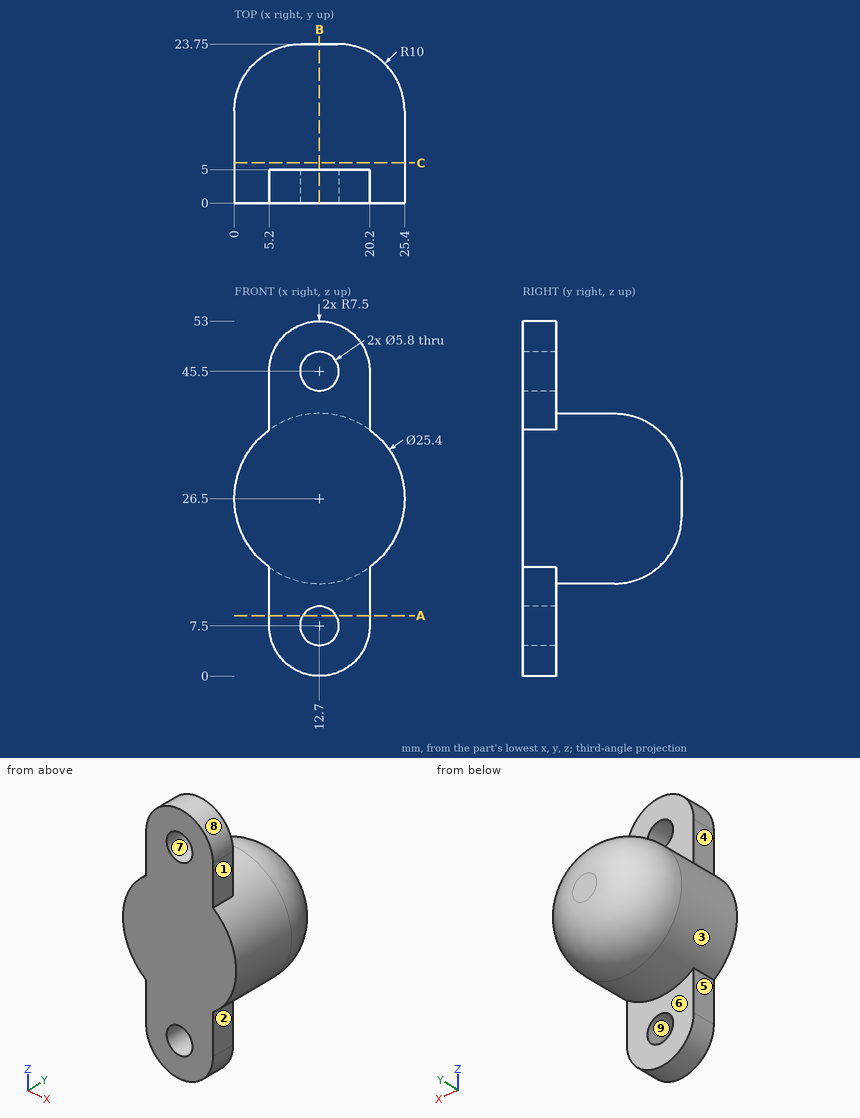
The drawing under review shows one solid part. Ordinate dimensions are in mm from its lowest x, y, z. A direction names the side the tool comes from. Coordinates: 2 decimals unless noted, no trailing zeros. Loops run counter-clockwise (first coordinate to the right, second up) from the corner with the lowest first, then second, coordinate; pieces in that order, holes last. Notation, with made-up numbers: (38, 41.5) - (63, 41.5) arc R12 cw to (63, 46.5) - close; hole circle Ø8 at (73, -40). An arc over 180 degrees is marked (long way). Return JSON: item names as keys, results as strings.
Item 1: Insertion check: pin 1 (5.5 mm diameter, centred on y = 2.5, z = 11, fed in from -X); pin 2 (8 mm diameter, centred on x = 20.5, y = 6, fed in from +Z); pin 3 (4 mm diameter, centred on x = 16, y = 5.5, fed in from +Z) (3 decimals). Each pin has a flat end and moves straight along its axis. Give the tip position at first contact, or say it passes through.
Determined:
{"pin 1": "stops at x = 5.2", "pin 2": "stops at z = 51.89", "pin 3": "stops at z = 52.875"}
Item 2: Take a section at A-A (z = 9). Give the boundary of the cut face in (x, y), then the cut area to 3 significant figures.
Determined:
{"outline": "(5.2, 0) - (10.22, 0) - (10.22, 5) - (5.2, 5) - close; (15.18, 0) - (20.2, 0) - (20.2, 5) - (15.18, 5) - close", "area": "50.2 mm2"}
Item 3: Mouldability with a two-part tool opening along X and no side actions: class the marked faces 6, 7, 8 and 9 as pulls with the +X half, pulls with the -X half, needs draft (parallel to the pull), parting line crosses it, or undercut.
Determined:
{"face 6": "needs draft", "face 7": "undercut", "face 8": "parting line crosses it", "face 9": "undercut"}
Item 4: For line 1 (X direction, y = 1.35, z = 7.5); line 2 (Y direction, x = 7.75, z = 45); line 3 (Z direction, x = 3, y = 20), list the stretches that pass through material, from the lowest coordinate up.
Determined:
{"line 1": "x = 5.2 to 9.8, 15.6 to 20.2", "line 2": "y = 0 to 5", "line 3": "z = 22.46 to 30.54"}
Item 5: Take a section at C-C (y = 6). Give the boundary of the cut face in (x, z), then the cut area to 3 significant figures.
Determined:
{"outline": "circle Ø25.4 at (12.7, 26.5)", "area": "507 mm2"}
Item 6: Take a section at B-B (x = 12.7). State how many separate pieces and enclosed holes the cut face has, then the cut area to 3 significant figures.
Determined:
{"separate pieces": "3", "enclosed holes": "0", "area": "640 mm2"}
Item 7: For the marked faces 1, 2, 3, 4 and 5, list the 3-axis set-ups (+Z, -Z, +X, -X, +Y, -Y) from which the entire face can be reached by the end or side of a thin tool; tool diameter is ignored.
Determined:
{"face 1": "+Z, +X, +Y, -Y", "face 2": "-Z, +X, +Y, -Y", "face 3": "+Y", "face 4": "+Z, -X, +Y, -Y", "face 5": "-Z, -X, +Y, -Y"}
